The figure shows three views and two pictorial views of one solid part (mm, origin at its lowest corner). Answer the questions. Coordinates: 2 decimals unless noted, no trailing zeros. Order: outer loops, then holes, each group sorted by start corner. A loop starts at its lowest first (then second) coordinate and runs counter-clockwise, first axis right, second up. Notation, with made-up numbers: (67, -34) -> (114, -34) arc R32 cw to (114, -3) -> close; hole circle Ø5 at (50, -20.75). An arc over 180 degrees is marked (long way). Return JSON: item names as keys, results as strings.
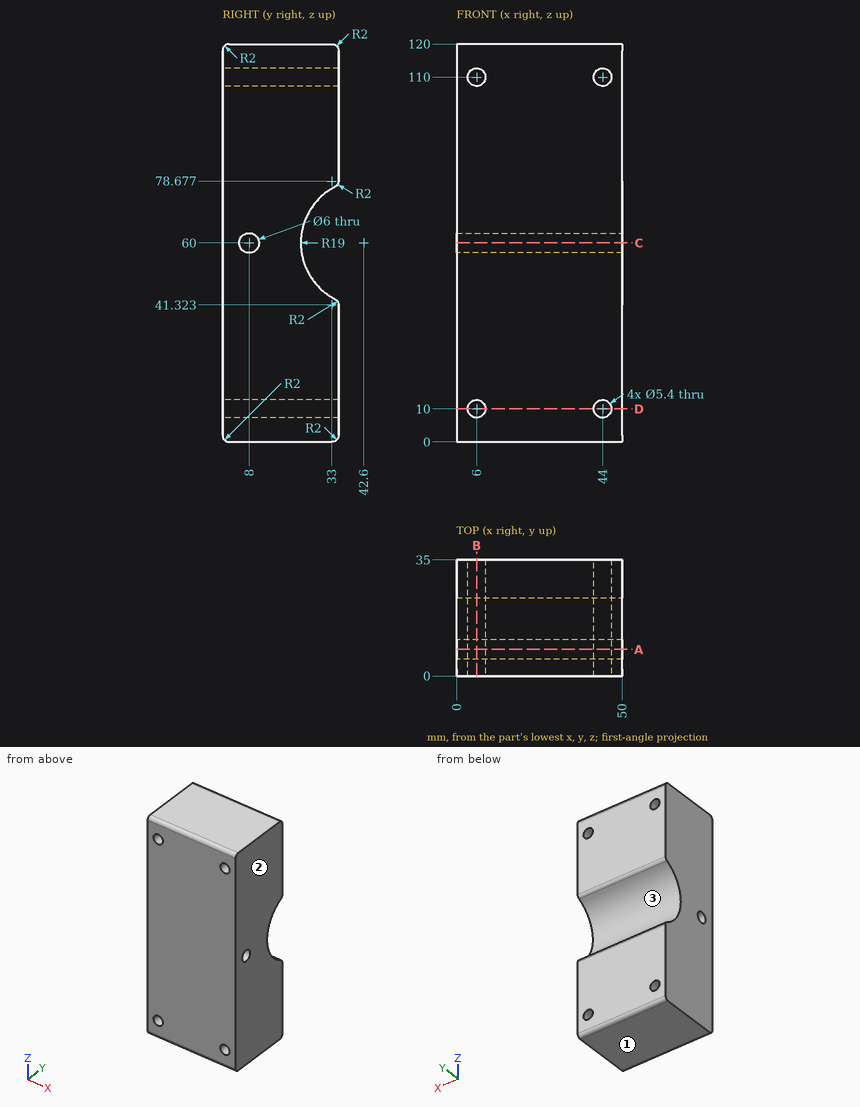
1. The part is cut by section D-D on z = 10. Give the vertices of the cut face in (x, y), and give its area (3 significant figures).
Answer block:
{"outline": "(0, 0) -> (3.3, 0) -> (3.3, 35) -> (0, 35) -> close; (8.7, 0) -> (41.3, 0) -> (41.3, 35) -> (8.7, 35) -> close; (46.7, 0) -> (50, 0) -> (50, 35) -> (46.7, 35) -> close", "area": "1,370 mm2"}
2. The part is cut by section C-C on z = 60. Give the vertices of the cut face in (x, y), and give its area (3 significant figures).
Answer block:
{"outline": "(0, 0) -> (50, 0) -> (50, 5) -> (0, 5) -> close; (0, 11) -> (50, 11) -> (50, 23.6) -> (0, 23.6) -> close", "area": "880 mm2"}
3. The part is cut by section B-B on x = 6. Give the vertices of the cut face in (y, z), and give its area (3 significant figures).
Answer block:
{"outline": "(0, 2) arc R2 ccw to (2, 0) -> (33, 0) arc R2 ccw to (35, 2) -> (35, 7.3) -> (0, 7.3) -> close; (0, 12.7) -> (35, 12.7) -> (35, 41.32) arc R2 ccw to (33.91, 43.1) arc R19 cw to (33.91, 76.9) arc R2 ccw to (35, 78.68) -> (35, 107.3) -> (0, 107.3) -> close; (0, 112.7) -> (35, 112.7) -> (35, 118) arc R2 ccw to (33, 120) -> (2, 120) arc R2 ccw to (0, 118) -> close; hole circle Ø6 at (8, 60)", "area": "3,500 mm2"}
4. Consider line 1 (Z direction, x = 44, y = 20); line 2 (Z direction, x = 6, y = 27) (1 decimal); line 3 (Z direction, x = 8, y = 3.5) (1 decimal). Determine where each line is inside the solid, lowest interval first. Write a range as from..to.
Answer block:
{"line 1": "z = 0..7.3, 12.7..107.3, 112.7..120", "line 2": "z = 0..7.3, 12.7..49.2, 70.8..107.3, 112.7..120", "line 3": "z = 0..8.2, 11.8..108.2, 111.8..120"}
5. Determine the mould class of the marked faces 1, 2 and 3 for opening direction Z: pulls with the +Z half, pulls with the -Z half, needs draft (parallel to the pull), parting line crosses it, or undercut.
Answer block:
{"face 1": "pulls with the -Z half", "face 2": "needs draft", "face 3": "undercut"}
6. The part is cut by section A-A on y = 8. Give the vertices of the cut face in (x, z), and give its area (3 significant figures).
Answer block:
{"outline": "(0, 0) -> (50, 0) -> (50, 57) -> (0, 57) -> close; (0, 63) -> (50, 63) -> (50, 120) -> (0, 120) -> close; hole circle Ø5.4 at (6, 10); hole circle Ø5.4 at (6, 110); hole circle Ø5.4 at (44, 10); hole circle Ø5.4 at (44, 110)", "area": "5,610 mm2"}
7. Each of these flat-tipped pins is pushed along its axis until it touches: pin 1 Ø5 at (x, y) = (23.5, 19) entering from -Z; pin 2 Ø12 at (x, z) = (15, 60.5) entering from +Y. Where does it stop, or does it pass through?
Answer block:
{"pin 1": "stops at z = 0", "pin 2": "stops at y = 24.75"}
